```python
from build123d import *

# Parameters (mm, degrees)
SKETCH1_R           = 14.93
BOSS_EXTRUDE1_DEPTH = 5.16
SKETCH2_R           = 0.85
BOSS_EXTRUDE2_DEPTH = 2.94
FILLET2_R           = 0.7
FILLET4_R           = 0.7
SKETCH3_R           = 3.515
CUT_EXTRUDE1_DEPTH  = 1.5


with BuildPart() as part:
    # Sketch1 → Boss-Extrude1 (new body)
    with BuildSketch(Plane(origin=(0, 0, 0), x_dir=(1, 0, 0), z_dir=(0, 1, 0))):
        Circle(SKETCH1_R)
    extrude(amount=BOSS_EXTRUDE1_DEPTH)

    # Sketch2 → Boss-Extrude2 (add)
    with BuildSketch(Plane(origin=(0, 0, 0), x_dir=(1, 0, 0), z_dir=(0, 1, 0))):
        with BuildLine():
            Line((-14.184219953, -4.659700025), (-20.406728453, -2.514915627))
            ThreePointArc((-20.406728453, -2.514915627), (-22.2, 0), (-20.406728453, 2.514915627))
            Line((-20.406728453, 2.514915627), (-14.184219953, 4.659700025))
            ThreePointArc((-14.184219953, 4.659700025), (-14.93, 0), (-14.184219953, -4.659700025))
        make_face()
        with Locations((-17.68, 0)):
            Circle(SKETCH2_R, mode=Mode.SUBTRACT)
        with BuildLine():
            Line((14.184219953, 4.659700025), (20.406728453, 2.514915627))
            ThreePointArc((20.406728453, 2.514915627), (22.2, 0), (20.406728453, -2.514915627))
            Line((20.406728453, -2.514915627), (14.184219953, -4.659700025))
            ThreePointArc((14.184219953, -4.659700025), (14.93, 0), (14.184219953, 4.659700025))
        make_face()
        with Locations((17.68, 0)):
            Circle(SKETCH2_R, mode=Mode.SUBTRACT)
    extrude(amount=BOSS_EXTRUDE2_DEPTH)

    # Fillet2
    fillet2_edges = [part.edges().sort_by_distance(p)[0] for p in [
        (-14.93, 5.16, 0),
    ]]
    fillet(fillet2_edges, radius=FILLET2_R)

    # Fillet4
    fillet4_edges = [part.edges().sort_by_distance(p)[0] for p in [
        (-22.2, 2.94, 0),
        (-17.295474203, 2.94, 3.587307826),
        (-17.295474203, 2.94, -3.587307826),
        (17.295474203, 2.94, 3.587307826),
        (22.2, 2.94, 0),
        (17.295474203, 2.94, -3.587307826),
    ]]
    fillet(fillet4_edges, radius=FILLET4_R)

    # Sketch3 → Cut-Extrude1 (cut)
    with BuildSketch(Plane(origin=(0, 5.16, 0), x_dir=(1, 0, 0), z_dir=(0, 1, 0))):
        Circle(SKETCH3_R)
    extrude(amount=-CUT_EXTRUDE1_DEPTH, mode=Mode.SUBTRACT)


solid = part.part
```
Can you work these out from the model? Positions are in its coordinate system, mm. A direction names the side the tool comes from. Give positions to 0.01 mm unless a question says otherwise; leave off trailing zeros. Loops run counter-clockwise (first coordinate to the right, second up) from the corner with the lowest first, then second, coordinate; pieces in that order, holes last. Notation, with made-up numbers: M -39.75,-33 L -15.75,-33 A5 ccw -15.75,-26 Z; hole C 56,58.25 d9. An arc over 180 degrees is marked long. Use CSV: the item, a comma, the result in double quotes. Start each with the question number.
1. Imagine slicing it at B-B, the plane y = 1.6. Write out the boundary of the cut face in (x, z).
2. For P1, Ø3, axis at x = 10, y = 3, coming from the -Z side; P2, Ø1, axis at x = -7, y = 2.5, coming from the +Z side; P3, Ø1.5, axis at x = 14, y = 4, coming from the -Z side; P4, Ø5.5, axis at x = 0, z = 0, coming from the -Y side, each with a flat end and sliding along its axis, tell me the tip position at first contact or that it passes through.
3. Imagine slicing it at A-A, the plane z = 0. Write out the boundary of the cut face in (x, y) (3 decimals).
4. If we mould it in two halves opening along X, with no side actions, what happens to faces 3 (the face through (-17.27, 2.74, 3.373)), 4 (the face through (-0.76, 4.42, 3.43)), 5 (the face through (17, 2.94, 1))? For each: released by +X, released by -X, zero draft, split by the parting line, or undercut.
5. Imagine slicing it at C-C, the plane x = 0. Write out the boundary of the cut face in (y, z) (3 decimals).
6. If I drill on L1, parallel to X at y = 1.9, z = 0; L2, parallel to X at y = 4.3, z = 0 (3 decimals); L3, parallel to X at y = 2.85, z = -0.75, over which ranges is the centre line in solid material (lowest first)?
7. On a 3-axis mill with a long thin cutter (end or side, diameter ignored), from which of +Z, -Z, +X, -X, +Y, -Y can I reach the whole of each face in a straight line? I mean faces 1 (the face through (0, 3.66, 0)), 2 (the face through (0, 0, 0)). Say none if no direction works.
Response values:
1,outline,"M -20.41,-2.51 L -14.18,-4.66 A14.93 ccw 14.18,-4.66 L 20.41,-2.51 A2.66 ccw 20.41,2.51 L 14.18,4.66 A14.93 ccw -14.18,4.66 L -20.41,2.51 A2.66 ccw Z; hole C -17.68,0 d1.7; hole C 17.68,0 d1.7"
2,P1,"z = -12.27"
2,P2,"z = 13.44"
2,P3,"z = -6.88"
2,P4,"y = 0"
3,outline,"M -22.2,0 L -18.53,0 L -18.53,2.94 L -21.5,2.94 A0.7 ccw -22.2,2.24 Z; M -16.83,0 L 16.83,0 L 16.83,2.94 L 14.93,2.94 L 14.93,4.46 A0.7 ccw 14.23,5.16 L 3.515,5.16 L 3.515,3.66 L -3.515,3.66 L -3.515,5.16 L -14.23,5.16 A0.7 ccw -14.93,4.46 L -14.93,2.94 L -16.83,2.94 Z; M 18.53,0 L 22.2,0 L 22.2,2.24 A0.7 ccw 21.5,2.94 L 18.53,2.94 Z"
4,face 3,"released by -X"
4,face 4,"undercut"
4,face 5,"zero draft"
5,outline,"M 0,-14.93 L 4.46,-14.93 A0.7 ccw 5.16,-14.23 L 5.16,-3.515 L 3.66,-3.515 L 3.66,3.515 L 5.16,3.515 L 5.16,14.23 A0.7 ccw 4.46,14.93 L 0,14.93 Z"
6,L1,"-22.2 to -18.53, -16.83 to 16.83, 18.53 to 22.2"
6,L2,"-14.93 to -3.515, 3.515 to 14.93"
6,L3,"-21.72 to -18.08, -17.28 to 17.28, 18.08 to 21.72"
7,face 1,"+Y"
7,face 2,"+Z, -Z, +X, -X, -Y"
